Autodesk Inventor part; units mm, degrees
ref_plane "YZ Plane" through (0, 0, 0) normal (1, 0, 0) x (0, 1, 0)
ref_plane "XZ Plane" through (0, 0, 0) normal (0, 1, 0) x (-1, 0, 0)
ref_plane "XY Plane" through (0, 0, 0) normal (0, 0, 1) x (1, 0, 0)
sketch "Szkic1" plane through (0, 0, 0) normal (0, 1, 0) x (-1, 0, 0)
  circle A0 centre (0, 0) radius 10
  circle A1 centre (0, 0) radius 15
  dimension "d0" = 20
  dimension "d1" = 30
extrude "Wyciągnięcie proste1" add sketch "Szkic1" along normal blind 60
sketch "Szkic2" plane through (0, 0, 0) normal (0, -1, 0) x (1, 0, 0)
  line L0 (2.5, 36.2128) -> (-2.5, 36.2128)
  line L1 (-2.5, 36.2128) -> (-2.5, 11.2128)
  line L2 (-2.5, 11.2128) -> (2.5, 11.2128)
  line L3 (2.5, 11.2128) -> (2.5, 36.2128)
  line L4 (2.5, 36.2128) -> (-2.5, 11.2128) construction
  line L5 (-2.5, 36.2128) -> (2.5, 11.2128) construction
  point P0 (0, 0)
  point P1 (0, 23.7128)
  dimension "d4" = 5
  dimension "d5" = 25
extrude "Wyciągnięcie proste2" add sketch "Szkic2" against normal blind 50
chamfer "Faza1" distance 21 distance2 49 1 edges at (0, 50, 36.2128) measured on face at (-0.2789, 50, 29.1341)
pattern_circular "Szyk kołowy1" count 3 over 360 about axis through (0, 0, 0) along (0, 1, 0) of "Faza1", "Wyciągnięcie proste2"
sketch "Szkic3" plane through (0, 0, 0) normal (0, -1, 0) x (1, 0, 0)
  arc A0 (-11.5587, -9.5602) -> (11.5587, -9.5602) centre (0, 0) ccw
  line L0 (11.5587, -9.5602) -> (30.1112, -20.2715)
  line L1 (30.1112, -20.2715) -> (32.6112, -15.9413)
  line L2 (32.6112, -15.9413) -> (14.0587, -5.23)
  arc A1 (14.0587, -5.23) -> (2.5, 14.7902) centre (0, 0) ccw
  line L3 (2.5, 14.7902) -> (2.5, 36.2128)
  line L4 (2.5, 36.2128) -> (-2.5, 36.2128)
  line L5 (-2.5, 36.2128) -> (-2.5, 14.7902)
  arc A2 (-2.5, 14.7902) -> (-14.0587, -5.23) centre (0, 0) ccw
  line L6 (-14.0587, -5.23) -> (-32.6112, -15.9413)
  line L7 (-32.6112, -15.9413) -> (-30.1112, -20.2715)
  line L8 (-30.1112, -20.2715) -> (-11.5587, -9.5602)
  circle A3 centre (0, 0) radius 10
  arc A4 (16.4473, -4.2997) -> (4.5, 16.3936) centre (0, 0) ccw
  line L9 (16.4473, -4.2997) -> (35.3433, -15.2093)
  line L10 (35.3433, -15.2093) -> (30.8433, -23.0035)
  line L11 (30.8433, -23.0035) -> (11.9473, -12.0939)
  arc A5 (-11.9473, -12.0939) -> (11.9473, -12.0939) centre (0, 0) ccw
  line L12 (-11.9473, -12.0939) -> (-30.8433, -23.0035)
  line L13 (-30.8433, -23.0035) -> (-35.3433, -15.2093)
  line L14 (-35.3433, -15.2093) -> (-16.4473, -4.2997)
  arc A6 (-4.5, 16.3936) -> (-16.4473, -4.2997) centre (0, 0) ccw
  line L15 (-4.5, 16.3936) -> (-4.5, 38.2128)
  line L16 (-4.5, 38.2128) -> (4.5, 38.2128)
  line L17 (4.5, 38.2128) -> (4.5, 16.3936)
  dimension "d14" = 2
extrude "Wyciągnięcie proste3" add sketch "Szkic3" along normal blind 2 contours L8 L7 L6 A2 L5 L4 L3 A1 L2 L1 L0 A0 | A3 | L9 L10 L11 A5 L12 L13 L14 A6 L15 L16 L17 A4
fillet "Zaokrąglenie1" radius 2 6 edges at (35.3433, -1, -15.2093) (30.8433, -1, -23.0035) (-30.8433, -1, -23.0035) (-35.3433, -1, -15.2093) (-4.5, -1, 38.2128) (4.5, -1, 38.2128)
chamfer "Faza2" distance 1 angle 45 2 edges at (15, 60, 0) (10, 60, 0)
properties part number "stojak" material "Polietylen, o małej gęstości"
Design review of the part built by this model. Coordinates are the model's own, in mm. A direction names the side the tool comes from. Coordinates: 2 decimals unless noted, no trailing zeros. Order: outer loops, then holes, each group sorted by start corner. A loop starts at its lowest first (then second) coordinate and runs counter-clockwise, first axis right, second up.
Item 1: For pin 1 Ø3 at (y, z) = (28, 18.5) entering from +X; pin 2 Ø1.5 at (x, y) = (8, 35.5) entering from -Z; pin 3 Ø2.5 at (x, z) = (-12.5, -6.5) entering from +Y; pin 4 Ø6.5 at (y, z) = (15.5, 24.5) entering from -X, all flat-tipped, find the tip position at first contact; note any pin that passes through.
Item 2: Take a section at D-D, the plane y = 25. Write out the cut boundary in (x, z).
Item 3: For line 1 (Z direction, x = 0, y = 40.5); line 2 (X direction, y = 43, z = -2); line 3 (Z direction, x = 0, y = 25.5), list the stretches that pass through material, from the lowest coordinate up.
Item 4: Take a section at B-B, the plane y = 42.5. Write out the cut boundary in (x, z).
Item 5: For faces 1 (the cylindrical face through (14.985, 29.087, -0.66)), 2 (the flat face through (-20.41, -0.99, -16.98)), 3 (the flat face through (-4.5, -1, 26)), 4 (the flat face through (-18.9, 19.1, -13.8)), list the 3-axis set-ups (+Z, -Z, +X, -X, +Y, -Y) from which the entire face can be reached by the end or side of a thin tool; tool diameter is ignored.
Item 6: Take a section at A-A, the plane x = 0. Write out the cut boundary in (y, z), then the cut area to 3 significant figures.
Item 7: The part is to be moulded in two halves that separate along Z. For faces 5 (the flat face through (0, 0, 0)), 6 (the flat face through (-6.2, 60, -9.3)), 7 (the cylindrical face through (-30.65, -1.014, -22.197)), say which applies: pulls with the +Z half, pulls with the -Z half, needs draft (parallel to the pull), parting line crosses it, or undercut.
Item 8: Take a section at C-C, the plane z = 0. Write out the cut boundary in (x, y).
The answers:
1. pin 1: stops at x = 2.5
1. pin 2: stops at z = -13.13
1. pin 3: stops at y = 60
1. pin 4: stops at x = -2.5
2. outline: (-23.7, -10.8) - (-21.2, -15.13) - (-11.56, -9.56) arc R15 ccw to (11.56, -9.56) - (21.2, -15.13) - (23.7, -10.8) - (14.06, -5.23) arc R15 ccw to (2.5, 14.79) - (2.5, 25.93) - (-2.5, 25.93) - (-2.5, 14.79) arc R15 ccw to (-14.06, -5.23) - close; hole circle Ø20 at (0, 0)
3. line 1: z = -15 to -10, 10 to 19.28
3. line 2: x = -14.87 to -9.8, 9.8 to 14.87
3. line 3: z = -15 to -10, 10 to 25.71
4. outline: (-17.21, -7.05) - (-14.71, -11.38) - (-11.56, -9.56) arc R15 ccw to (11.56, -9.56) - (14.71, -11.38) - (17.21, -7.05) - (14.06, -5.23) arc R15 ccw to (2.5, 14.79) - (2.5, 18.43) - (-2.5, 18.43) - (-2.5, 14.79) arc R15 ccw to (-14.06, -5.23) - close; hole circle Ø20 at (0, 0)
5. face 1: +Y
5. face 2: -Z, +Y, -Y
5. face 3: +Z, -X, +Y, -Y
5. face 4: -Z, +Y
6. outline: (-2, -17) - (0, -17) - (0, -15) - (59, -15) - (60, -14) - (60, -11) - (59, -10) - (0, -10) - (0, 10) - (59, 10) - (60, 11) - (60, 14) - (59, 15) - (50, 15) - (50, 15.21) - (1, 36.21) - (0, 36.21) - (0, 38.21) - (-2, 38.21) - close
6. area: 1,250 mm2
7. face 5: undercut
7. face 6: needs draft
7. face 7: pulls with the -Z half
8. outline: (-17, -2) - (17, -2) - (17, 0) - (15, 0) - (15, 59) - (14, 60) - (11, 60) - (10, 59) - (10, 0) - (-10, 0) - (-10, 59) - (-11, 60) - (-14, 60) - (-15, 59) - (-15, 0) - (-17, 0) - close
